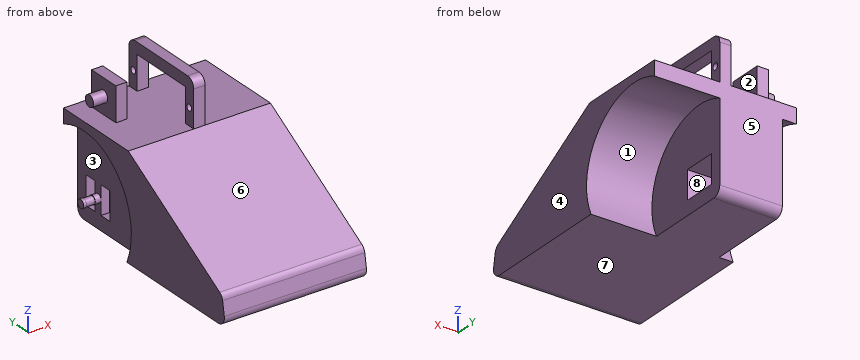
from build123d import *

# Parameters (mm, degrees)
F1_DEPTH  = 23
F0_W      = 12
F0_H      = 10
F2_DEPTH  = 19
F3_W      = 3
F3_H      = 10
F4_DEPTH  = 3
F6_DEPTH  = 2
F7_R      = 1.35
F8_DEPTH  = 3.1
F9_R      = 1.5
F9_R_2    = 1.35
F10_DEPTH = 1
F12_DEPTH = 5
F0_R      = 1.15
F13_DEPTH = 4
F16_DEPTH = 4
F17_R     = 2
F18_DEPTH = 5


with BuildPart() as f1:
    # F0 (on Right) → F1 (new body)
    with BuildSketch(Plane.YZ):
        with BuildLine():
            Line((12, -6), (-12, -6))
            Line((-12, -6), (-16, -6))
            Line((-16, -6), (-25.9322462259, -11.7637196141))
            Line((-25.9322462259, -11.7637196141), (-47.8941944105, -24.5083202449))
            Line((-47.8941944105, -24.5083202449), (-61.0953553653, -32.1690032962))
            ThreePointArc((-61.0953553653, -32.1690032962), (-62.0489693843, -33.0457447692), (-62.5440346563, -34.2428102162))
            Line((-62.5440346563, -34.2428102162), (-63.3791624813, -38.979055467))
            ThreePointArc((-63.3791624813, -38.979055467), (-62.7228725516, -41.4283628291), (-60.4247392222, -42.5))
            Line((-60.4247392222, -42.5), (-15.2661703181, -42.5))
            ThreePointArc((-15.2661703181, -42.5), (-10.6170093579, -15.8829906421), (16, -11.2338296819))
            Line((16, -11.2338296819), (16, -6))
            Line((16, -6), (12, -6))
        make_face()
    extrude(amount=F1_DEPTH)

    # F0 (on Right) → F2 (join)
    with BuildSketch(Plane.YZ):
        with BuildLine():
            Line((16, -39.5), (16, -11.2338296819))
            ThreePointArc((16, -11.2338296819), (-10.6170093579, -15.8829906421), (-15.2661703181, -42.5))
            Line((-15.2661703181, -42.5), (13, -42.5))
            ThreePointArc((13, -42.5), (15.1213203436, -41.6213203436), (16, -39.5))
        make_face()
        with Locations((6, -32.5)):
            Rectangle(F0_W, F0_H, mode=Mode.SUBTRACT)
        with BuildLine():
            Line((12, -6), (-12, -6))
            Line((-12, -6), (-16, -6))
            Line((-16, -6), (-25.9322462259, -11.7637196141))
            Line((-25.9322462259, -11.7637196141), (-47.8941944105, -24.5083202449))
            Line((-47.8941944105, -24.5083202449), (-61.0953553653, -32.1690032962))
            ThreePointArc((-61.0953553653, -32.1690032962), (-62.0489693843, -33.0457447692), (-62.5440346563, -34.2428102162))
            Line((-62.5440346563, -34.2428102162), (-63.3791624813, -38.979055467))
            ThreePointArc((-63.3791624813, -38.979055467), (-62.7228725516, -41.4283628291), (-60.4247392222, -42.5))
            Line((-60.4247392222, -42.5), (-15.2661703181, -42.5))
            ThreePointArc((-15.2661703181, -42.5), (-10.6170093579, -15.8829906421), (16, -11.2338296819))
            Line((16, -11.2338296819), (16, -6))
            Line((16, -6), (12, -6))
        make_face()
    extrude(amount=-F2_DEPTH)

    # F3 (on face) → F4 (join)
    with BuildSketch(Plane(origin=(-19, 0, 0), x_dir=(0, -1, 0), z_dir=(-1, 0, 0))):
        with BuildLine():
            Line((-16, -6), (-16, -39.5))
            ThreePointArc((-16, -39.5), (-15.1213203436, -41.6213203436), (-13, -42.5))
            Line((-13, -42.5), (60.4247392222, -42.5))
            ThreePointArc((60.4247392222, -42.5), (62.7228725516, -41.4283628291), (63.3791624813, -38.979055467))
            Line((63.3791624813, -38.979055467), (62.5440346563, -34.2428102162))
            ThreePointArc((62.5440346563, -34.2428102162), (62.0489693843, -33.0457447692), (61.0953553653, -32.1690032962))
            Line((61.0953553653, -32.1690032962), (16, -6))
            Line((16, -6), (-16, -6))
        make_face()
        Polygon((-12, -27.5), (-7.5, -27.5), (-4.5, -27.5), (0, -27.5), (0, -37.5), (-4.5, -37.5), (-7.5, -37.5), (-12, -37.5), align=None, mode=Mode.SUBTRACT)
        with Locations((-6, -32.5)):
            Rectangle(F3_W, F3_H)
    extrude(amount=F4_DEPTH)

    # F5 (on face) → F6 (join)
    with BuildSketch(Plane(origin=(-22, 0, 0), x_dir=(0, -1, 0), z_dir=(-1, 0, 0))):
        with BuildLine():
            ThreePointArc((-7.5, -32.5), (-6, -34), (-4.5, -32.5))
            ThreePointArc((-4.5, -32.5), (-6, -31), (-7.5, -32.5))
        make_face()
    extrude(amount=F6_DEPTH)

    # F7 (on face) → F8 (join)
    with BuildSketch(Plane(origin=(-24, 0, 0), x_dir=(0, -1, 0), z_dir=(-1, 0, 0))):
        with Locations((-6, -32.5)):
            Circle(F7_R)
    extrude(amount=F8_DEPTH)

    # F9 (on face) → F10 (join)
    with BuildSketch(Plane(origin=(-27.1, 0, 0), x_dir=(0, -1, 0), z_dir=(-1, 0, 0))):
        with Locations((-6, -32.5)):
            Circle(F9_R)
        with Locations((-6, -32.5)):
            Circle(F9_R_2, mode=Mode.SUBTRACT)
        with Locations((-6, -32.5)):
            Circle(F9_R_2)
    extrude(amount=F10_DEPTH)

    # F11 (on face) → F12 (join)
    with BuildSketch(Plane(origin=(-22, 0, 0), x_dir=(0, -1, 0), z_dir=(-1, 0, 0))):
        with BuildLine():
            ThreePointArc((-16, -11.2419736034), (10.6117983114, -15.8882016886), (15.2580263966, -42.5))
            Line((15.2580263966, -42.5), (60.4247392222, -42.5))
            ThreePointArc((60.4247392222, -42.5), (62.7228725516, -41.4283628291), (63.3791624813, -38.979055467))
            Line((63.3791624813, -38.979055467), (62.5440346563, -34.2428102162))
            ThreePointArc((62.5440346563, -34.2428102162), (62.0489693843, -33.0457447692), (61.0953553653, -32.1690032962))
            Line((61.0953553653, -32.1690032962), (16, -6))
            Line((16, -6), (-16, -6))
            Line((-16, -6), (-16, -11.2419736034))
        make_face()
    extrude(amount=F12_DEPTH)

    # F0 (on Right) → F13 (join)
    with BuildSketch(Plane.YZ):
        with BuildLine():
            Line((-12, -6), (-12, 6))
            Line((-12, 6), (12, 6))
            Line((12, 6), (12, -6))
            Line((12, -6), (16, -6))
            Line((16, -6), (16, 7))
            ThreePointArc((16, 7), (15.1213203436, 9.1213203436), (13, 10))
            Line((13, 10), (0, 10))
            Line((0, 10), (-13, 10))
            ThreePointArc((-13, 10), (-15.1213203436, 9.1213203436), (-16, 7))
            Line((-16, 7), (-16, -6))
            Line((-16, -6), (-12, -6))
        make_face()
        with Locations((-13.8, 0)):
            Circle(F0_R, mode=Mode.SUBTRACT)
        with Locations((13.8, 0)):
            Circle(F0_R, mode=Mode.SUBTRACT)
    extrude(amount=-F13_DEPTH)

    # F15 (on offset) → F16 (join)
    with BuildSketch(Plane.YZ.offset(-16)):
        Polygon((0, -6), (12, -6), (12, 0), (12, 6), (0, 6), align=None)
    extrude(amount=-F16_DEPTH)

    # F17 (on face) → F18 (join)
    with BuildSketch(Plane(origin=(-20, 0, 0), x_dir=(0, -1, 0), z_dir=(-1, 0, 0))):
        with Locations((-6, 0)):
            Circle(F17_R)
    extrude(amount=F18_DEPTH)


solid = f1.part
Can you work these out from the model? Positions are in its coordinate system, mm. Face numbers are marked on the shaded views. A direction names the side the tool comes from. Round coordinates to 2 decimals unless told otherwise and drop trailing zeros. Loops run counter-clockwise (first coordinate to the right, second up) from the corner with the lowest first, then second, coordinate; pieces in that order, holes last. Notation, with made-up numbers: (-38, 11.25) - (-14, 11.25) arc R15 ccw to (-14, 35.25) - close; hole circle Ø8 at (61, 29). An arc over 180 degrees is marked (long way). Answer in a Markdown table with one row per item. Add a question column.
Q1. I want a section at C-C on z = -18.5. List the corners of the cut face in (x, y) for me, and give its area (3 significant figures).
Q2. I want a section at B-B on x = -7. List the corners of the cut face in (y, z) for me.
Q3. Which directions (+Z, -Z, +X, -X, +Y, -Y) give clear straight access to the entire face, cutting with the end or side of a thin tool? Please do the marked faces 1, 2, 3 and 4.
Q4. I want a section at A-A on z = 0. List the corners of the cut face in (x, y) for me.
Q5. I want a section at D-D on x = 3. List the corners of the cut face in (y, z) for me, and give its area (3 significant figures).
Q6. I need wall thicknesses on L1, parallel to X at y = -8, z = -36; L2, parallel to Z at x = -1.6, y = 13.8; L3, parallel to X at y = -38, z = -39. Which ranges of each line are inside material? Lowest first, please.
Q7. We'd pull the mould along Z, two halves only. Please class the marked faces 5, 6, 7 and 8: pulls with the +Z half, pulls with the -Z half, needs draft (parallel to the pull), parting line crosses it, or undercut.
Q8. For pin 1 Ø12 at (y, z) = (-41.5, -28.5) entering from -X; pin 2 Ø3 at (x, z) = (-6, -31) entering from -Y; pin 3 Ø1.2 at (x, z) = (-2, 2) entering from -Y; pin 4 Ø13 at (y, z) = (4.5, 0) entering from +X, each with a flat end and sliding along its axis, tell me the tip position at first contact or that it passes through.
A:
| question | item | result |
|---|---|---|
| 1 | outline | (-27, -37.54) - (23, -37.54) - (23, -12.87) - (0, -12.87) - (0, 16) - (-22, 16) - (-22, -12.87) - (-27, -12.87) - close |
| 1 | area | 1,870 mm^2 |
| 2 | outline | (-63.38, -38.98) arc R3 ccw to (-60.42, -42.5) - (13, -42.5) arc R3 ccw to (16, -39.5) - (16, -6) - (-16, -6) - (-61.1, -32.17) arc R3 ccw to (-62.54, -34.24) - close; hole (0, -37.5) - (12, -37.5) - (12, -27.5) - (0, -27.5) - close |
| 3 | face 1 | +X |
| 3 | face 2 | +Z, +X, +Y, -Y |
| 3 | face 3 | -X |
| 3 | face 4 | +Z, -Z, +X, +Y, -Y |
| 4 | outline | (-25, 4) - (-20, 4) - (-20, 0) - (-16, 0) - (-16, 12) - (-20, 12) - (-20, 8) - (-25, 8) - close; (-4, -16) - (0, -16) - (0, -14.95) - (-4, -14.95) - close; (-4, -12.65) - (0, -12.65) - (0, -12) - (-4, -12) - close; (-4, 12) - (0, 12) - (0, 12.65) - (-4, 12.65) - close; (-4, 14.95) - (0, 14.95) - (0, 16) - (-4, 16) - close |
| 5 | outline | (-63.38, -38.98) arc R3 ccw to (-60.42, -42.5) - (-15.27, -42.5) arc R23.5 cw to (16, -11.23) - (16, -6) - (-16, -6) - (-61.1, -32.17) arc R3 ccw to (-62.54, -34.24) - close |
| 5 | area | 1,250 mm^2 |
| 6 | L1 | -22 to 0 |
| 6 | L2 | -42.39 to -1.15, 1.15 to 9.89 |
| 6 | L3 | -27 to 23 |
| 7 | face 5 | needs draft |
| 7 | face 6 | pulls with the +Z half |
| 7 | face 7 | pulls with the -Z half |
| 7 | face 8 | undercut |
| 8 | pin 1 | x = -27 |
| 8 | pin 2 | y = -61.56 |
| 8 | pin 3 | y = -16 |
| 8 | pin 4 | x = 23 |
